```python
from build123d import *

# Parameters (mm, degrees)
F0_R     = 30
F1_DEPTH = 100
F2_R     = 28
F3_DEPTH = 98
F4_W     = 10
F4_H     = 20
F5_DEPTH = 30


with BuildPart() as f1:
    # F0 (on Top) → F1 (new body)
    with BuildSketch(Plane.XY):
        Circle(F0_R)
    extrude(amount=F1_DEPTH)

    # F2 (on face) → F3 (cut)
    with BuildSketch(Plane.XY.offset(100)):
        Circle(F2_R)
    extrude(amount=-F3_DEPTH, mode=Mode.SUBTRACT)

    # F4 (on Front) → F5 (cut)
    with BuildSketch(Plane.XZ):
        with Locations((0, 80)):
            Rectangle(F4_W, F4_H)
    extrude(amount=F5_DEPTH, mode=Mode.SUBTRACT)


solid = f1.part
```
Source: CAD feature listing. Evaluate the final solid. Frame: model axes, mm. A direction names the side the tool comes from. Coordinates: 2 decimals unless noted, no trailing zeros. Write each loop counter-clockwise with the first axis right and the second up, starting at its lowest first coordinate (ties: lowest second). Pieces come first, ordered by that corner, then holes. Notation, with made-up numbers: (-31.75, -16) - (9.25, -16) arc R9 ccw to (9.25, -4) - close; hole circle Ø10 at (69.5, 82). An arc over 180 degrees is marked (long way). Answer as a JSON object with one key per item and string values.
Q1. Section query B-B, the plane y = 0. Output: boundary loops of the cut face in (x, z).
Ans:
{"outline": "(-30, 0) - (30, 0) - (30, 100) - (28, 100) - (28, 2) - (-28, 2) - (-28, 100) - (-30, 100) - close"}
Q2. Draft query along Z for faces 4 (the flat face through (0, 0, 0)), 5 (the flat face through (0, 0, 2)), 6 (the flat face through (-5, -29, 80)), 7 (the flat face through (0, -29, 90)). Return one class per face: released by +Z, released by -Z, zero draft, split by the parting line, or undercut.
Ans:
{"face 4": "released by -Z", "face 5": "released by +Z", "face 6": "undercut", "face 7": "undercut"}
Q3. Material intervals for line 1 (Z direction, x = -20, y = -19.5); line 2 (Y direction, x = 0, z = 67); line 3 (Y direction, x = 19, z = 92.5), sorted ascending. Write a range as [from, to].
Ans:
{"line 1": "z = [0, 2]", "line 2": "y = [-30, -28], [28, 30]", "line 3": "y = [-23.22, -20.57], [20.57, 23.22]"}
Q4. First-contact query: pin 1 Ø1.5 at (x, y) = (-4, 2.5) entering from +Z; pin 2 Ø12 at (y, z) = (-6.5, 87) entering from +X; pin 3 Ø1.5 at (x, z) = (-3, 52) entering from +Y; pin 4 Ø3 at (x, y) = (6, 16) entering from -Z. Flat tips, straight axial feed; report the tip coordinate or a pass-through.
Ans:
{"pin 1": "stops at z = 2", "pin 2": "stops at x = 30", "pin 3": "stops at y = 29.92", "pin 4": "stops at z = 0"}
Q5. Section query A-A, the plane x = 0. Output: boundary loops of the cut face in (y, z).
Ans:
{"outline": "(-30, 0) - (30, 0) - (30, 100) - (28, 100) - (28, 2) - (-28, 2) - (-28, 70) - (-30, 70) - close; (-30, 90) - (-28, 90) - (-28, 100) - (-30, 100) - close"}
Q6. Set-up query: faces 1 (the flat face through (5, -29, 80)), 2 (the flat face through (-25, 13, 100)), 3 (the cylindrical face through (25.865, -10.724, 51.686)). Return all of +Z, -Z, +X, -X, +Y, -Y with unobstructed straight access to the full face (end or side cutting, diameter ignored); none if empty.
Ans:
{"face 1": "-Y", "face 2": "+Z, +X, -X, +Y, -Y", "face 3": "+Z"}
Q7. Section query C-C, the plane x = 10. Output: boundary loops of the cut face in (y, z), plus the area to 3 significant figures.
Ans:
{"outline": "(-28.28, 0) - (28.28, 0) - (28.28, 100) - (26.15, 100) - (26.15, 2) - (-26.15, 2) - (-26.15, 100) - (-28.28, 100) - close", "area": "531 mm2"}
Q8. Section query D-D, the plane z = 78. Output: boundary loops of the cut face in (x, y).
Ans:
{"outline": "(-5, -29.58) - (-5, -27.55) arc R28 cw (long way) to (5, -27.55) - (5, -29.58) arc R30 ccw (long way) to start"}
